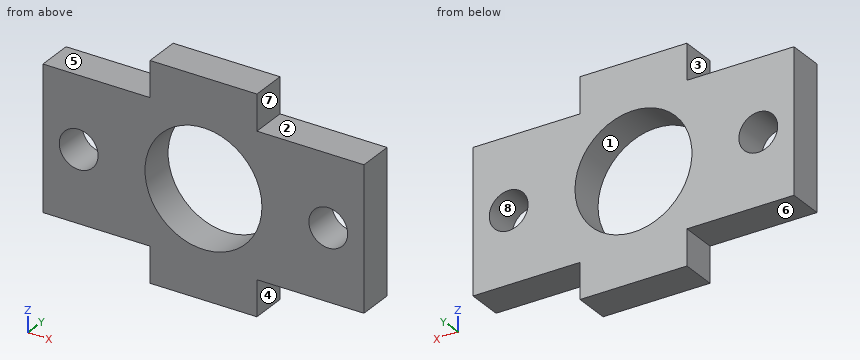
from build123d import *

# Parameters (mm, degrees)
SKETCH1_W           = 57.15
SKETCH1_H           = 25.4
SKETCH1_R           = 10.414
SKETCH1_R_2         = 3.4544
BOSS_EXTRUDE1_DEPTH = 6.35
SKETCH2_W           = 19.05
SKETCH2_H           = 6.35
BOSS_EXTRUDE2_DEPTH = 6.35


with BuildPart() as part:
    # Sketch1 → Boss-Extrude1 (new body)
    with BuildSketch(Plane(origin=(0, 0, 0), x_dir=(1, 0, 0), z_dir=(0, 1, 0))):
        Rectangle(SKETCH1_W, SKETCH1_H)
        Circle(SKETCH1_R, mode=Mode.SUBTRACT)
        with Locations((-22.225, 0)):
            Circle(SKETCH1_R_2, mode=Mode.SUBTRACT)
        with Locations((22.225, 0)):
            Circle(SKETCH1_R_2, mode=Mode.SUBTRACT)
    extrude(amount=BOSS_EXTRUDE1_DEPTH)

    # Sketch2 → Boss-Extrude2 (add)
    with BuildSketch(Plane(origin=(0, 6.35, 0), x_dir=(1, 0, 0), z_dir=(0, 1, 0))):
        with Locations((0, 15.875)):
            Rectangle(SKETCH2_W, SKETCH2_H)
    boss_extrude2 = extrude(amount=-BOSS_EXTRUDE2_DEPTH)

    # Mirror1: Boss-Extrude2 across plane
    add(boss_extrude2.mirror(Plane.XY))


solid = part.part
Can you work these out from the model? Positions are in its coordinate system, mm. Face numbers are marked on the shaded views. A direction names the side the tool comes from. Coordinates: 2 decimals unless noted, no trailing zeros. Write each loop counter-clockwise with the first axis right and the second up, starting at its lowest first coordinate (ties: lowest second). Pieces come first, ordered by that corner, then holes. Notation, with made-up numbers: (43.5, 32.5) -> (49.5, 32.5) arc R19 ccw to (49.5, 47.5) -> close; hole circle Ø3 at (-12, 82.5). An arc over 180 degrees is marked (long way). Answer as CSV lines item,"result".
1) Will these pins go through, and if not, where does the flat tip stop? P1, Ø1.9, axis at y = 2.5, z = -15.5, coming from the +X side (3 decimals); P2, Ø1.9, axis at y = 4.5, z = 17, coming from the -X side (3 decimals); P3, Ø3, axis at x = 17, y = 4.5, coming from the +Z side; P4, Ø12.5, axis at x = 0, z = 0, coming from the +Y side.
Check result:
P1,"x = 9.525"
P2,"x = -9.525"
P3,"z = 12.7"
P4,"through"
2) If I drill on line 1 (X direction, y = 2.25, z = 0) (3 decimals); line 2 (X direction, y = 5.5, z = -1) (1 decimal); line 3 (Z direction, x = 22, y = 4.75), over which ranges is the centre line in solid material (lowest first)? Write a range as from..to.
Check result:
line 1,"-28.575..-25.679, -18.771..-10.414, 10.414..18.771, 25.679..28.575"
line 2,"-28.6..-25.5, -18.9..-10.4, 10.4..18.9, 25.5..28.6"
line 3,"-12.7..-3.45, 3.45..12.7"
3) If we section it at D-D on z = 7.5: Please give me the cut outline in (x, y) (3 decimals).
Check result:
outline,"(-28.575, 0) -> (-7.225, 0) -> (-7.225, 6.35) -> (-28.575, 6.35) -> close; (7.225, 0) -> (28.575, 0) -> (28.575, 6.35) -> (7.225, 6.35) -> close"
4) If we section it at B-B on x = 0: Please give me the cut outline in (y, z), then the cut area to 3 significant figures.
Check result:
outline,"(0, -19.05) -> (6.35, -19.05) -> (6.35, -10.41) -> (0, -10.41) -> close; (0, 10.41) -> (6.35, 10.41) -> (6.35, 19.05) -> (0, 19.05) -> close"
area,"110 mm²"
5) On a 3-axis mill with a long thin cutter (end or side, diameter ignored), from which of +Z, -Z, +X, -X, +Y, -Y can I reach the whole of each face in a straight line? I mean the marked faces 4, 5, 6, 7 and 8. Say none if no direction works.
Check result:
face 4,"-Z, +X, +Y, -Y"
face 5,"+Z, -X, +Y, -Y"
face 6,"-Z, -X, +Y, -Y"
face 7,"+Z, +X, +Y, -Y"
face 8,"+Y, -Y"
6) If we section it at C-C on y = 2.5: Please give me the cut outline in (x, z) (3 decimals), then the cut area to 3 significant figures.
Check result:
outline,"(-28.575, -12.7) -> (-9.525, -12.7) -> (-9.525, -19.05) -> (9.525, -19.05) -> (9.525, -12.7) -> (28.575, -12.7) -> (28.575, 12.7) -> (9.525, 12.7) -> (9.525, 19.05) -> (-9.525, 19.05) -> (-9.525, 12.7) -> (-28.575, 12.7) -> close; hole circle Ø6.909 at (-22.225, 0); hole circle Ø20.828 at (0, 0); hole circle Ø6.909 at (22.225, 0)"
area,"1,280 mm²"
7) If we mould it in two halves opening along X, with no side actions, what happens to the marked faces 1, 2 and 3? For each: +X half, -X half, draft (parallel to the pull), parting line (faces both ways), or undercut.
Check result:
face 1,"undercut"
face 2,"draft"
face 3,"-X half"
8) If we section it at A-A on z = 0: Please give me the cut outline in (x, y) (3 decimals), then the cut area to 3 significant figures.
Check result:
outline,"(-28.575, 0) -> (-25.679, 0) -> (-25.679, 6.35) -> (-28.575, 6.35) -> close; (-18.771, 0) -> (-10.414, 0) -> (-10.414, 6.35) -> (-18.771, 6.35) -> close; (10.414, 0) -> (18.771, 0) -> (18.771, 6.35) -> (10.414, 6.35) -> close; (25.679, 0) -> (28.575, 0) -> (28.575, 6.35) -> (25.679, 6.35) -> close"
area,"143 mm²"
